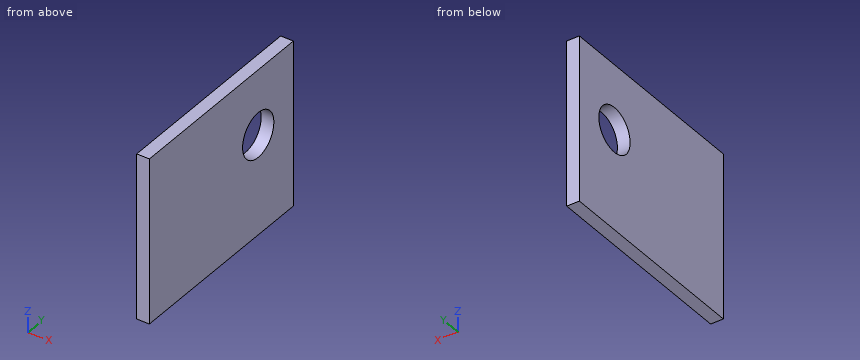
from build123d import *

# Parameters (mm, degrees)
CROQUIS2_W              = 244
CROQUIS2_H              = 195
CROQUIS2_R              = 26.5
SALIENTE_EXTRUIR1_DEPTH = 15


with BuildPart() as part:
    # Croquis2 → Saliente-Extruir1 (new body)
    with BuildSketch(Plane.YZ):
        with Locations((122, 97.5)):
            Rectangle(CROQUIS2_W, CROQUIS2_H)
        with Locations(Location((184.5, 118, 0), (0, 0, 270))):
            Circle(CROQUIS2_R, mode=Mode.SUBTRACT)
    extrude(amount=SALIENTE_EXTRUIR1_DEPTH)


solid = part.part
Geometry: final body of the model. Coordinates: model frame, mm. Coordinates: 2 decimals unless noted, no trailing zeros. Loops run counter-clockwise (first coordinate to the right, second up) from the corner with the lowest first, then second, coordinate; pieces in that order, holes last. Notation, with made-up numbers: M -13.5,55.5 L 9.5,55.5 A28 ccw 9.5,82.5 Z; hole C 73.25,26.25 d5. An arc over 180 degrees is marked long. One line per item, written item: value. Start each with the question number.
1) Cut plane C-C (x = 8). Return loops of the section in (y, z), then the cut area to 3 significant figures.
2) Cut plane B-B (z = 118). Return loops of the section in (x, y), then the cut area to 4 significant figures.
3) Cut plane A-A (y = 184.5). Return loops of the section in (x, z).
4) Material intervals for L1, parallel to Y at x = 10.5, z = 118; L2, parallel to Y at x = 13.5, z = 110; L3, parallel to Z at x = 1, y = 191.5, sorted ascending. Write a range as from..to.
Evaluation:
1. outline: M 0,0 L 244,0 L 244,195 L 0,195 Z; hole C 184.5,118 d53
1. area: 45,400 mm^2
2. outline: M 0,0 L 15,0 L 15,158 L 0,158 Z; M 0,211 L 15,211 L 15,244 L 0,244 Z
2. area: 2,865 mm^2
3. outline: M 0,0 L 15,0 L 15,91.5 L 0,91.5 Z; M 0,144.5 L 15,144.5 L 15,195 L 0,195 Z
4. L1: 0..158, 211..244
4. L2: 0..159.24, 209.76..244
4. L3: 0..92.44, 143.56..195
